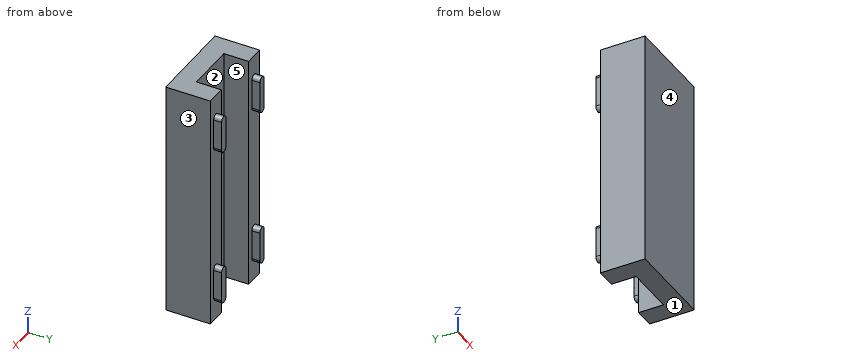
from build123d import *

# Parameters (mm, degrees)
BOSS_EXTRUDE1_DEPTH     = 120
CUT_EXTRUDE1_DEPTH      = 2.5
CUT_EXTRUDE1_DEPTH_BACK = 2.5
BOSS_EXTRUDE2_DEPTH     = 4
MIRROR2_COPY_1_DEPTH    = 4


with BuildPart() as part:
    # Sketch1 → Boss-Extrude1 (new body)
    with BuildSketch(Plane.XY):
        Polygon((-12.5, 12.5), (-22.5, 12.5), (-22.5, -10), (22.5, -10), (22.5, 12.5), (12.5, 12.5), (12.5, 0), (-12.5, 0), align=None)
    extrude(amount=BOSS_EXTRUDE1_DEPTH)

    # Sketch2 → Cut-Extrude1 (cut, two sides: drawn at the far end of the back side and taken through both)
    with BuildSketch(Plane(origin=(0, 0, 0), x_dir=(0, 0, -1), z_dir=(1, 0, 0)).offset(-CUT_EXTRUDE1_DEPTH_BACK)):
        Polygon((-29.416511254, 0), (-99.416511254, 0), (-99.416511254, -6.5), align=None)
    extrude(amount=CUT_EXTRUDE1_DEPTH + CUT_EXTRUDE1_DEPTH_BACK, mode=Mode.SUBTRACT)

    # Sketch3 → Boss-Extrude2 (add)
    with BuildSketch(Plane(origin=(0, 12.5, 0), x_dir=(1, 0, 0), z_dir=(0, 1, 0))):
        with BuildLine():
            Line((-19.5, -108), (-19.5, -93))
            ThreePointArc((-19.5, -93), (-17.5, -91), (-15.5, -93))
            Line((-15.5, -93), (-15.5, -108))
            ThreePointArc((-15.5, -108), (-17.5, -110), (-19.5, -108))
        make_face()
    boss_extrude2 = extrude(amount=BOSS_EXTRUDE2_DEPTH)

    # Mirror1: Boss-Extrude2 across plane
    add(boss_extrude2.mirror(Plane(origin=(0, 0, 0), x_dir=(0, 0, 1), z_dir=(1, 0, 0))))

    # Mirror2: Boss-Extrude2 across plane
    add(boss_extrude2.mirror(Plane(origin=(0, 0, 60), x_dir=(1, 0, 0), z_dir=(0, 0, -1))))

    # Mirror2 copy 1 sketch → Mirror2 copy 1 (add)
    with BuildSketch(Plane(origin=(0, 12.5, 120), x_dir=(-1, 0, 0), z_dir=(0, 1, 0))):
        with BuildLine():
            Line((-19.5, -108), (-19.5, -93))
            ThreePointArc((-19.5, -93), (-17.5, -91), (-15.5, -93))
            Line((-15.5, -93), (-15.5, -108))
            ThreePointArc((-15.5, -108), (-17.5, -110), (-19.5, -108))
        make_face()
    extrude(amount=MIRROR2_COPY_1_DEPTH)


solid = part.part
Build history of the part. All positions in model axes, mm. Face numbers are marked on the shaded views. A direction names the side the tool comes from. Coordinates: 2 decimals unless noted, no trailing zeros. Write each loop counter-clockwise with the first axis right and the second up, starting at its lowest first coordinate (ties: lowest second). Pieces come first, ordered by that corner, then holes. Notation, with made-up numbers: (7, 57) -> (43, 57) arc R17 cw to (43, 84) -> close; hole circle Ø8 at (-9, 36.25). An arc over 180 degrees is marked (long way). Use CSV: the item, a comma, the result in double quotes. Start each with the question number.
Q1. Cut at B-B, the plane z = 8. List the corners of the cut face in (x, y), then the cut area to 3 significant figures.
Q2. Pull direction X, two halves, no side cores. Call the marked faces 3, 4 and 5: released by +X, released by -X, zero draft, split by the parting line, or undercut.
Q3. Flat gauge pins, fed straight in: pin 1 Ø3 at (y, z) = (15, 99) entering from -X; pin 2 Ø8 at (x, z) = (17.5, 60.5) entering from +Y; pin 3 Ø1.2 at (y, z) = (13.5, 17) entering from +X. Where does each tip first touch, or does it go through?
Q4. Cut at D-D, the plane z = 102. List the corners of the cut face in (x, y), then the cut area to 3 significant figures.
Q5. Cut at A-A, the plane y = 10.25. List the corners of the cut face in (x, z).
Q6. Drill centre lines: probe 1 along X at (y, z) = (7.75, 53); probe 2 along X at (y, z) = (13.25, 93.5); probe 3 along Y at (x, z) = (-3.5, 53). Where is each one in solid material? Low to high.
Q7. Cut at C-C, the plane x = 17.5. List the corners of the cut face in (y, z).
Q8. 3-axis set-ups, long thin cutter, end or side, ignore diameter. For the marked faces 1 and 2: which of +Z, -Z, +X, -X, +Y, -Y reach the whole face in a straight line?
Checked values:
1,outline,"(-22.5, -10) -> (22.5, -10) -> (22.5, 12.5) -> (12.5, 12.5) -> (12.5, 0) -> (-12.5, 0) -> (-12.5, 12.5) -> (-22.5, 12.5) -> close"
1,area,"700 mm²"
2,face 3,"released by +X"
2,face 4,"zero draft"
2,face 5,"undercut"
3,pin 1,"stops at x = -19.5"
3,pin 2,"stops at y = 12.5"
3,pin 3,"stops at x = 19.5"
4,outline,"(-22.5, -10) -> (22.5, -10) -> (22.5, 12.5) -> (19.5, 12.5) -> (19.5, 16.5) -> (15.5, 16.5) -> (15.5, 12.5) -> (12.5, 12.5) -> (12.5, 0) -> (-12.5, 0) -> (-12.5, 12.5) -> (-15.5, 12.5) -> (-15.5, 16.5) -> (-19.5, 16.5) -> (-19.5, 12.5) -> (-22.5, 12.5) -> close"
4,area,"732 mm²"
5,outline,"(-22.5, 0) -> (-12.5, 0) -> (-12.5, 120) -> (-22.5, 120) -> close; (12.5, 0) -> (22.5, 0) -> (22.5, 120) -> (12.5, 120) -> close"
6,probe 1,"x = -22.5 to -12.5, 12.5 to 22.5"
6,probe 2,"x = -19.5 to -15.5, 15.5 to 19.5"
6,probe 3,"y = -10 to 0"
7,outline,"(-10, 0) -> (12.5, 0) -> (12.5, 10) -> (16.5, 10) -> (16.5, 29) -> (12.5, 29) -> (12.5, 91) -> (16.5, 91) -> (16.5, 110) -> (12.5, 110) -> (12.5, 120) -> (-10, 120) -> close"
8,face 1,"-Z, +X, -X, +Y, -Y"
8,face 2,"+Z, -Z, +Y"
